from build123d import *

# Parameters (mm, degrees)
EXTRUDE_THIN1_DEPTH         = 609.6
F_1_4_CLEARANCE_HOLE1_D     = 6.7564
F_1_4_CLEARANCE_HOLE1_DEPTH = 25.4
F_1_4_CLEARANCE_HOLE1_TIP   = 2.029827343


with BuildPart() as part:
    # Sketch1 → Extrude-Thin1 (new, symmetric)
    with BuildSketch(Plane.XY):
        with BuildLine():
            Line((-12.5, -10), (-12.5, 10))
            ThreePointArc((-12.5, 10), (-11.767766953, 11.767766953), (-10, 12.5))
            Line((-10, 12.5), (10, 12.5))
            ThreePointArc((10, 12.5), (11.767766953, 11.767766953), (12.5, 10))
            Line((12.5, 10), (12.5, -10))
            ThreePointArc((12.5, -10), (11.767766953, -11.767766953), (10, -12.5))
            Line((10, -12.5), (-10, -12.5))
            ThreePointArc((-10, -12.5), (-11.767766953, -11.767766953), (-12.5, -10))
        make_face()
        with BuildLine():
            Line((-10.5, -10), (-10.5, 10))
            ThreePointArc((-10.5, 10), (-10.353553391, 10.353553391), (-10, 10.5))
            Line((-10, 10.5), (10, 10.5))
            ThreePointArc((10, 10.5), (10.353553391, 10.353553391), (10.5, 10))
            Line((10.5, 10), (10.5, -10))
            ThreePointArc((10.5, -10), (10.353553391, -10.353553391), (10, -10.5))
            Line((10, -10.5), (-10, -10.5))
            ThreePointArc((-10, -10.5), (-10.353553391, -10.353553391), (-10.5, -10))
        make_face(mode=Mode.SUBTRACT)
    extrude(amount=EXTRUDE_THIN1_DEPTH, both=True)

    # 1/4 Clearance Hole1
    with Locations(Plane(origin=(0, 12.5, 0), x_dir=(1, 0, 0), z_dir=(0, 1, 0))):
        with Locations((-0.2, 596.9), (-0.2, -596.9)):
            Hole(F_1_4_CLEARANCE_HOLE1_D / 2, depth=F_1_4_CLEARANCE_HOLE1_DEPTH)
            with Locations((0, 0, -(F_1_4_CLEARANCE_HOLE1_DEPTH + F_1_4_CLEARANCE_HOLE1_TIP / 2))):  # 118° drill point
                Cone(0, F_1_4_CLEARANCE_HOLE1_D / 2, F_1_4_CLEARANCE_HOLE1_TIP, mode=Mode.SUBTRACT)


solid = part.part
Part model, mm, in its own coordinate system. A direction names the side the tool comes from. Give positions to 0.01 mm unless a question says otherwise; leave off trailing zeros. Loops run counter-clockwise (first coordinate to the right, second up) from the corner with the lowest first, then second, coordinate; pieces in that order, holes last. Notation, with made-up numbers: M 76,54 L 120,54 A31 ccw 120,89 Z; hole C -19.75,62.25 d1. An arc over 180 degrees is marked long. Put each result on its own line as item: value. Start each with the question number.
1) Pull direction X, two halves, no side cores. Call faces 3 (the flat face through (0, -10.5, 9)), 4 (the flat face through (11, 0, -609.6)), 5 (the flat face through (12.5, 0, 9)): +X half, -X half, draft (parallel to the pull), parting line (faces both ways), or undercut.
2) Saw through at A-A (z = 194.5). List the corners of the cut face in (x, y).
3) 3-axis set-ups, long thin cutter, end or side, ignore diameter. For faces 1 (the flat face through (0, -12.5, 9)), 2 (the flat face through (10.5, 0, 9)): which of +Z, -Z, +X, -X, +Y, -Y reach the whole face in a straight line?
4) Probe probe 1 along Z at (x, y) = (-0.2, 11.35); probe 2 along Y at (x, z) = (-8.5, 136.5). List the from-to ranges inside material, lowest first.
Numbers:
1. face 3: undercut
1. face 4: draft
1. face 5: +X half
2. outline: M -12.5,-10 A2.5 ccw -10,-12.5 L 10,-12.5 A2.5 ccw 12.5,-10 L 12.5,10 A2.5 ccw 10,12.5 L -10,12.5 A2.5 ccw -12.5,10 Z; hole M -10.5,-10 A0.5 ccw -10,-10.5 L 10,-10.5 A0.5 ccw 10.5,-10 L 10.5,10 A0.5 ccw 10,10.5 L -10,10.5 A0.5 ccw -10.5,10 Z
3. face 1: +Z, -Z, +X, -X, -Y
3. face 2: +Z, -Z
4. probe 1: -609.6 to -600.28, -593.52 to 593.52, 600.28 to 609.6
4. probe 2: -12.5 to -10.5, 10.5 to 12.5
